The listing builds one solid part. Answer for the finished solid, in the listing's coordinates (mm). Round coordinates to 2 decimals unless told otherwise and drop trailing zeros. Order: outer loops, then holes, each group sorted by start corner. A loop starts at its lowest first (then second) coordinate and runs counter-clockwise, first axis right, second up. Notation, with made-up numbers: M 59,61 L 89,61 A31 cw 89,85 Z; hole C 6,20.25 d4. An arc over 180 degrees is marked long. Put each result on its own line as item: value. Start each with the question number.
1. The mould has two halves that part along Y. Classify faces 1 (the face through (-4, 5, -4.5)), 2 (the face through (-2, 6, -2.5)), 3 (the face through (-1.172, 8.923, -0.049)): +Y half, -Y half, draft (parallel to the pull), parting line (faces both ways), or undercut.
2. The part is cut by section C-C (z = -3). Give the vertices of the cut face in (x, y), then the cut area to 3 significant figures.
3. Each of these flat-tipped pins is pushed along its axis until it touches: pin 1 Ø8 at (x, y) = (-5.5, 1) entering from +Z; pin 2 Ø6 at (x, y) = (2, -3) entering from +Z; pin 3 Ø1.5 at (y, z) = (-4.5, 0.5) entering from -X. Where does it stop, or does it pass through?
4. Consider line 1 (Y direction, x = 0, z = 1.25); line 2 (Y direction, x = 0, z = -3.15); line 3 (X direction, y = 2.75, z = 3.25). Determine where each line is inside the solid, lowest interval first.
5. The part is cut by section D-D (z = 3.25). Give the vertices of the cut face in (x, y).
from build123d import *

# Parameters (mm, degrees)
SKETCH1_R           = 10
SKETCH1_R_2         = 9
SKETCH1_R_3         = 7.1
BOSS_EXTRUDE1_DEPTH = 4.5
SKETCH1_3_R         = 10
SKETCH1_3_R_2       = 9
CUT_EXTRUDE1_DEPTH  = 3.5
CHAMFER1_SIZE       = 1
SKETCH2_R           = 7.1
SKETCH2_R_2         = 6.1
BOSS_EXTRUDE2_DEPTH = 2


with BuildPart() as part:
    # Sketch1 → Boss-Extrude1 (new, symmetric)
    # profile 1 of 2: a face of its own
    with BuildSketch(Plane.XY):
        Circle(SKETCH1_R)
        Circle(SKETCH1_R_2, mode=Mode.SUBTRACT)
    # profile 2 of 2: a face of its own
    with BuildSketch(Plane.XY):
        Circle(SKETCH1_R_2)
        Circle(SKETCH1_R_3, mode=Mode.SUBTRACT)
    extrude(amount=BOSS_EXTRUDE1_DEPTH, both=True)

    # Sketch1<3> → Cut-Extrude1 (cut, symmetric)
    with BuildSketch(Plane.XY):
        Circle(SKETCH1_3_R)
        Circle(SKETCH1_3_R_2, mode=Mode.SUBTRACT)
    extrude(amount=CUT_EXTRUDE1_DEPTH, both=True, mode=Mode.SUBTRACT)

    # Chamfer1
    chamfer1_edges = [part.edges().sort_by_distance(p)[0] for p in [
        (-10, 0, -3.5),
        (-10, 0, 3.5),
    ]]
    chamfer(chamfer1_edges, length=CHAMFER1_SIZE - 0.0001)  # a hair under: the kernel refuses the full size

    # Sketch2 → Boss-Extrude2 (add)
    with BuildSketch(Plane(origin=(0, 0, -4.5), x_dir=(-1, 0, 0), z_dir=(0, 0, -1))):
        Circle(SKETCH2_R)
        Circle(SKETCH2_R_2, mode=Mode.SUBTRACT)
    extrude(amount=-BOSS_EXTRUDE2_DEPTH)


solid = part.part
Resolved:
1. face 1: draft
1. face 2: undercut
1. face 3: parting line
2. outline: C 0,0 d18; hole C 0,0 d12.2
2. area: 138 mm2
3. pin 1: z = 4.5
3. pin 2: z = -2.5
3. pin 3: x = -8.18
4. line 1: -9 to -7.1, 7.1 to 9
4. line 2: -9 to -6.1, 6.1 to 9
4. line 3: -8.57 to -6.55, 6.55 to 8.57
5. outline: C 0,0 d18; hole C 0,0 d14.2
